Read the model definition and answer for the solid it produces. Units are mm, in the model's axes. A direction names the side the tool comes from. Round coordinates to 2 decimals unless told otherwise and drop trailing zeros. Order: outer loops, then holes, each group sorted by start corner. A loop starts at its lowest first (then second) coordinate and runs counter-clockwise, first axis right, second up.
from build123d import *

# Parameters (mm, degrees)
SKETCH2_W           = 50
SKETCH2_H           = 55
SKETCH2_R           = 1.65
BOSS_EXTRUDE2_DEPTH = 6
SKETCH4_R           = 3
SKETCH4_R_2         = 1.65
BOSS_EXTRUDE3_DEPTH = 3.5
SKETCH5_R           = 3
CUT_EXTRUDE2_DEPTH  = 3
SKETCH6_W           = 50
SKETCH6_H           = 3.75
SKETCH6_H_2         = 6
CUT_EXTRUDE3_DEPTH  = 10
SKETCH7_W           = 50
SKETCH7_H           = 45.25
CUT_EXTRUDE4_DEPTH  = 1


with BuildPart() as part:
    # Sketch2 → Boss-Extrude2 (new body)
    with BuildSketch(Plane(origin=(0, 0, 0), x_dir=(1, 0, 0), z_dir=(0, 1, 0))):
        with Locations((25, 27.5)):
            Rectangle(SKETCH2_W, SKETCH2_H)
        with Locations((6, 10)):
            Circle(SKETCH2_R, mode=Mode.SUBTRACT)
        with Locations((44, 10)):
            Circle(SKETCH2_R, mode=Mode.SUBTRACT)
        with Locations((44, 48)):
            Circle(SKETCH2_R, mode=Mode.SUBTRACT)
        with Locations((6, 48)):
            Circle(SKETCH2_R, mode=Mode.SUBTRACT)
        with Locations((6, 29)):
            Circle(SKETCH2_R, mode=Mode.SUBTRACT)
        with Locations((44, 29)):
            Circle(SKETCH2_R, mode=Mode.SUBTRACT)
    extrude(amount=BOSS_EXTRUDE2_DEPTH)

    # Sketch4 → Boss-Extrude3 (add)
    with BuildSketch(Plane(origin=(0, 6, 0), x_dir=(1, 0, 0), z_dir=(0, 1, 0))):
        with Locations((6, 10)):
            Circle(SKETCH4_R)
        with Locations((6, 10)):
            Circle(SKETCH4_R_2, mode=Mode.SUBTRACT)
        with Locations((44, 10)):
            Circle(SKETCH4_R)
        with Locations((44, 10)):
            Circle(SKETCH4_R_2, mode=Mode.SUBTRACT)
        with Locations((6, 48)):
            Circle(SKETCH4_R)
        with Locations((6, 48)):
            Circle(SKETCH4_R_2, mode=Mode.SUBTRACT)
        with Locations((44, 48)):
            Circle(SKETCH4_R)
        with Locations((44, 48)):
            Circle(SKETCH4_R_2, mode=Mode.SUBTRACT)
    extrude(amount=BOSS_EXTRUDE3_DEPTH)

    # Sketch5 → Cut-Extrude2 (cut)
    with BuildSketch(Plane(origin=(0, 6, 0), x_dir=(1, 0, 0), z_dir=(0, 1, 0))):
        with Locations((6, 29)):
            Circle(SKETCH5_R)
        with Locations((44, 29)):
            Circle(SKETCH5_R)
    extrude(amount=-CUT_EXTRUDE2_DEPTH, mode=Mode.SUBTRACT)

    # Sketch6 → Cut-Extrude3 (cut)
    with BuildSketch(Plane(origin=(0, 6, 0), x_dir=(1, 0, 0), z_dir=(0, 1, 0))):
        with Locations((25, 53.125)):
            Rectangle(SKETCH6_W, SKETCH6_H)
        with Locations((25, 3)):
            Rectangle(SKETCH6_W, SKETCH6_H_2)
    extrude(amount=-CUT_EXTRUDE3_DEPTH, mode=Mode.SUBTRACT)

    # Sketch7 → Cut-Extrude4 (cut)
    with BuildSketch(Plane.XZ):
        with Locations((25, -28.625)):
            Rectangle(SKETCH7_W, SKETCH7_H)
    extrude(amount=-CUT_EXTRUDE4_DEPTH, mode=Mode.SUBTRACT)


solid = part.part
Q1. A cutting plane is placed at C-C, the plane x = 44. Give the vertices of the cut face in (y, z), plus the area to 3 significant figures.
Outcome:
outline: (1, -51.25) - (6, -51.25) - (6, -51) - (9.5, -51) - (9.5, -49.65) - (1, -49.65) - close; (1, -46.35) - (9.5, -46.35) - (9.5, -45) - (6, -45) - (6, -32) - (3, -32) - (3, -30.65) - (1, -30.65) - close; (1, -27.35) - (3, -27.35) - (3, -26) - (6, -26) - (6, -13) - (9.5, -13) - (9.5, -11.65) - (1, -11.65) - close; (1, -8.35) - (9.5, -8.35) - (9.5, -7) - (6, -7) - (6, -6) - (1, -6) - close
area: 188 mm2
Q2. For faces 1 (the face through (7.3, 3, -27.7)), 2 (the face through (50, 3, -28)), determine the directions among +Z, -Z, +X, -X, +Y, -Y from which every point of the face is accessible in a straight line to the end or side of a thin tool.
Outcome:
face 1: +Y
face 2: +Z, -Z, +X, +Y, -Y
Q3. A cutting plane is placed at A-A, the plane y = 7.5. Give the vertices of the cut face in (x, z).
Outcome:
outline: circle Ø6 at (6, -48); circle Ø6 at (6, -10); circle Ø6 at (44, -48); circle Ø6 at (44, -10); hole circle Ø3.3 at (6, -48); hole circle Ø3.3 at (6, -10); hole circle Ø3.3 at (44, -48); hole circle Ø3.3 at (44, -10)
Q4. For a pull along Z with two mould halves and no side action, classify faces 3 (the face through (42.35, 5.19, -10.07)), 4 (the face through (45.3, 9.5, -46.7)), 5 (the face through (25, 4, -6)) as released by +Z, released by -Z, zero draft, split by the parting line, or undercut.
Outcome:
face 3: undercut
face 4: zero draft
face 5: released by +Z
Q5. Flat-ended cylindrical pins translate along their axes: pin 1 (13.5 mm diameter, centred on x = 19.5, z = -18, fed in from +Y); pin 2 (4 mm diameter, centred on x = 6, z = -48, fed in from -Y). Find the tip coordinate at first contact, or state that the pin passes through.
Outcome:
pin 1: stops at y = 6
pin 2: stops at y = 1
Q6. A cutting plane is placed at D-D, the plane z = -29. Give the vertices of the cut face in (x, y).
Outcome:
outline: (0, 1) - (4.35, 1) - (4.35, 3) - (3, 3) - (3, 6) - (0, 6) - close; (7.65, 1) - (42.35, 1) - (42.35, 3) - (41, 3) - (41, 6) - (9, 6) - (9, 3) - (7.65, 3) - close; (45.65, 1) - (50, 1) - (50, 6) - (47, 6) - (47, 3) - (45.65, 3) - close
Q7. A cutting plane is placed at B-B, the plane z = -10. Give the vertices of the cut face in (x, y).
Outcome:
outline: (0, 1) - (4.35, 1) - (4.35, 9.5) - (3, 9.5) - (3, 6) - (0, 6) - close; (7.65, 1) - (42.35, 1) - (42.35, 9.5) - (41, 9.5) - (41, 6) - (9, 6) - (9, 9.5) - (7.65, 9.5) - close; (45.65, 1) - (50, 1) - (50, 6) - (47, 6) - (47, 9.5) - (45.65, 9.5) - close
Q8. Straight lines are drawn through the part: probe 1 along Z at (x, y) = (44, 6.5); probe 2 along X at (y, z) = (5.25, -29); probe 3 along X at (y, z) = (3.5, -48). For each, find the intervals that lie inside material, in ascending order.
Outcome:
probe 1: z = -51 to -49.65, -46.35 to -45, -13 to -11.65, -8.35 to -7
probe 2: x = 0 to 3, 9 to 41, 47 to 50
probe 3: x = 0 to 4.35, 7.65 to 42.35, 45.65 to 50
